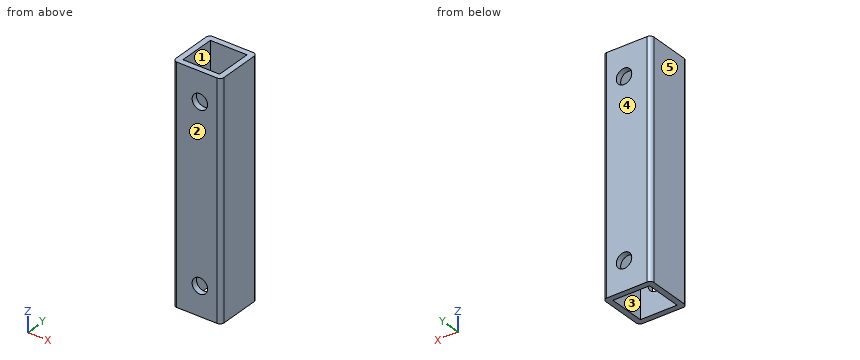
from build123d import *

# Parameters (mm, degrees)
EXTRUDE_THIN1_DEPTH      = 60
EXTRUDE_THIN1_DEPTH_BACK = 60
SKETCH1_W                = 25
SKETCH1_H                = 25
SKETCH1_W_2              = 19
SKETCH1_H_2              = 19
FILLET1_R                = 2
SKETCH3_R                = 4
CUT_EXTRUDE2_DEPTH       = 67.191011474


with BuildPart() as part:
    # Sketch1 → Extrude-Thin1 (new, two sides: drawn at the far end of the back side and taken through both)
    with BuildSketch(Plane.XY.offset(-EXTRUDE_THIN1_DEPTH_BACK)):
        Rectangle(SKETCH1_W, SKETCH1_H)
        Rectangle(SKETCH1_W_2, SKETCH1_H_2, mode=Mode.SUBTRACT)
    extrude(amount=EXTRUDE_THIN1_DEPTH + EXTRUDE_THIN1_DEPTH_BACK)

    # Fillet1
    fillet1_edges = [part.edges().sort_by_distance(p)[0] for p in [
        (12.5, -12.5, 0),
        (-12.5, -12.5, 0),
        (-12.5, 12.5, 0),
        (12.5, 12.5, 0),
    ]]
    fillet(fillet1_edges, radius=FILLET1_R)

    # Sketch3 → Cut-Extrude2 (cut, through all)
    with BuildSketch(Plane(origin=(0, 12.5, 0), x_dir=(1, 0, 0), z_dir=(0, 1, 0))):
        with Locations(Location((1.5, -45, 0), (0, 0, 270))):
            Circle(SKETCH3_R)
        with Locations(Location((1.5, 45, 0), (0, 0, 270))):
            Circle(SKETCH3_R)
    extrude(amount=-CUT_EXTRUDE2_DEPTH, mode=Mode.SUBTRACT)


solid = part.part
The listing builds one solid part. Answer for the finished solid, in the listing's coordinates (mm). Face numbers are marked on the shaded views. A direction names the side the tool comes from. Round coordinates to 2 decimals unless told otherwise and drop trailing zeros. Order: outer loops, then holes, each group sorted by start corner. A loop starts at its lowest first (then second) coordinate and runs counter-clockwise, first axis right, second up. Notation, with made-up numbers: (-13.5, -1.75) -> (38.5, -1.75) arc R13 cw to (38.5, 21.25) -> close; hole circle Ø5 at (4, -14.75). An arc over 180 degrees is marked (long way). Write each question's results on one line, items separated by ' | '. Start each with the question number.
Q1. Which of the six approach directions +Z, -Z, +X, -X, +Y, -Y give full straight-line access (tool end or side, diameter ignored) to the marked faces 1 and 2?
Q2. Find section D-D (z = -14.5). Determine the outline of the cut face in (x, y).
Q3. The mould has two halves that part along Y. Classify the marked faces 3, 4 and 5: pulls with the +Y half, pulls with the -Y half, needs draft (parallel to the pull), parting line crosses it, or undercut.
Q4. Find section B-B (x = -3.75). Determine the outline of the cut face in (y, z).
Q5. Find section A-A (z = -45). Determine the outline of the cut face in (x, y), then the cut area to 3 significant figures.
Q6. Straight lines are drawn through the part: probe 1 along X at (y, z) = (10.55, 45); probe 2 along Y at (x, z) = (-4.75, -6.5); probe 3 along Z at (x, y) = (2.25, 10.25). For each, find the intervals that lie inside material, in ascending order. Write a range as from..to.
Worked answers:
1) face 1: +Z, -Z | face 2: +Z, -Z, +X, -X, -Y
2) outline: (-12.5, -10.5) arc R2 ccw to (-10.5, -12.5) -> (10.5, -12.5) arc R2 ccw to (12.5, -10.5) -> (12.5, 10.5) arc R2 ccw to (10.5, 12.5) -> (-10.5, 12.5) arc R2 ccw to (-12.5, 10.5) -> close; hole (-9.5, -9.5) -> (9.5, -9.5) -> (9.5, 9.5) -> (-9.5, 9.5) -> close
3) face 3: undercut | face 4: pulls with the +Y half | face 5: needs draft
4) outline: (-12.5, -60) -> (-9.5, -60) -> (-9.5, 60) -> (-12.5, 60) -> close; (9.5, -60) -> (12.5, -60) -> (12.5, 60) -> (9.5, 60) -> close
5) outline: (-12.5, -10.5) arc R2 ccw to (-10.5, -12.5) -> (-2.5, -12.5) -> (-2.5, -9.5) -> (-9.5, -9.5) -> (-9.5, 9.5) -> (-2.5, 9.5) -> (-2.5, 12.5) -> (-10.5, 12.5) arc R2 ccw to (-12.5, 10.5) -> close; (5.5, -12.5) -> (10.5, -12.5) arc R2 ccw to (12.5, -10.5) -> (12.5, 10.5) arc R2 ccw to (10.5, 12.5) -> (5.5, 12.5) -> (5.5, 9.5) -> (9.5, 9.5) -> (9.5, -9.5) -> (5.5, -9.5) -> close | area: 213 mm2
6) probe 1: x = -12.5..-2.5, 5.5..12.5 | probe 2: y = -12.5..-9.5, 9.5..12.5 | probe 3: z = -60..-48.93, -41.07..41.07, 48.93..60
